Geometry: final body of the model. Coordinates: model frame, mm. A direction names the side the tool comes from. Give positions to 0.01 mm unless a question says otherwise; leave off trailing zeros. Write each loop counter-clockwise with the first axis right and the second up, starting at its lowest first coordinate (ties: lowest second). Pieces come first, ordered by that corner, then holes. Notation, with made-up numbers: (75.5, 89.5) - (101.5, 89.5) arc R13 cw to (101.5, 96.5) - close; hole circle Ø10 at (56.5, 62.5). An arc over 180 degrees is marked (long way). Return JSON: item names as keys, results as strings.
from build123d import *

# Parameters (mm, degrees)
SKETCH1_R           = 1.5
SKETCH1_W           = 23
SKETCH1_H           = 12
BOSS_EXTRUDE1_DEPTH = 5
FILLET1_R           = 5
FILLET2_R           = 5
FILLET3_R           = 5
FILLET4_R           = 5
FILLET5_R           = 5
FILLET6_R           = 5


with BuildPart() as part:
    # Sketch1 → Boss-Extrude1 (new body)
    with BuildSketch(Plane.XY):
        Polygon((28.231059773, 10.187376726), (15.644565305, 25.187376726), (-9.182445759, 25.187376726), (-21.768940227, 10.187376726), (-21.768940227, -14.812623274), (-16.768940227, -14.812623274), (-16.768940227, -9.812623274), (-11.768940227, -9.812623274), (-11.768940227, -14.812623274), (-4.768940227, -14.812623274), (-4.768940227, -9.812623274), (11.231059773, -9.812623274), (11.231059773, -14.812623274), (18.231059773, -14.812623274), (18.231059773, -9.812623274), (23.231059773, -9.812623274), (23.231059773, -14.812623274), (28.231059773, -14.812623274), align=None)
        with Locations((-2.768940227, 22.187376726)):
            Circle(SKETCH1_R, mode=Mode.SUBTRACT)
        with Locations((9.231059773, 22.187376726)):
            Circle(SKETCH1_R, mode=Mode.SUBTRACT)
        with Locations((-6.361893004, 3.645929715)):
            Circle(SKETCH1_R, mode=Mode.SUBTRACT)
        with Locations((11.531059773, 3.445929715)):
            Rectangle(SKETCH1_W, SKETCH1_H, mode=Mode.SUBTRACT)
    extrude(amount=BOSS_EXTRUDE1_DEPTH)

    # Fillet1
    fillet1_edges = [part.edges().sort_by_distance(p)[0] for p in [
        (15.644565305, 25.187376726, 2.5),
    ]]
    fillet(fillet1_edges, radius=FILLET1_R)

    # Fillet2
    fillet2_edges = [part.edges().sort_by_distance(p)[0] for p in [
        (28.231059773, 10.187376726, 2.5),
    ]]
    fillet(fillet2_edges, radius=FILLET2_R)

    # Fillet3
    fillet3_edges = [part.edges().sort_by_distance(p)[0] for p in [
        (28.231059773, -14.812623274, 2.5),
    ]]
    fillet(fillet3_edges, radius=FILLET3_R - 0.0001)  # a hair under: the kernel refuses the full size

    # Fillet4
    fillet4_edges = [part.edges().sort_by_distance(p)[0] for p in [
        (-9.182445759, 25.187376726, 2.5),
    ]]
    fillet(fillet4_edges, radius=FILLET4_R)

    # Fillet5
    fillet5_edges = [part.edges().sort_by_distance(p)[0] for p in [
        (-21.768940227, 10.187376726, 2.5),
    ]]
    fillet(fillet5_edges, radius=FILLET5_R)

    # Fillet6
    fillet6_edges = [part.edges().sort_by_distance(p)[0] for p in [
        (-21.768940227, -14.812623274, 2.5),
    ]]
    fillet(fillet6_edges, radius=FILLET6_R - 0.0001)  # a hair under: the kernel refuses the full size


solid = part.part
Q1. Section query B-B, the plane x = 6. Return the cut outline in (y, z).
Answer key:
{"outline": "(-9.81, 0) - (-2.55, 0) - (-2.55, 5) - (-9.81, 5) - close; (9.45, 0) - (25.19, 0) - (25.19, 5) - (9.45, 5) - close"}
Q2. Set-up query: faces 1 (the flat face through (-21.769, -1, 2)), 2 (the flat face through (11.231, -12, 2)), 3 (the flat face through (23.031, 3, 2)). Return all of +Z, -Z, +X, -X, +Y, -Y with unobstructed straight access to the full face (end or side cutting, diameter ignored); none if empty.
Answer key:
{"face 1": "+Z, -Z, -X, +Y, -Y", "face 2": "+Z, -Z, -Y", "face 3": "+Z, -Z"}
Q3. Mould query, pull axis X, two halves, no side actions, for faces 4 (the flat face through (15, -14.813, 2)), 5 (the cylindrical face through (27.92, 10.1, 2.54)), 6 (the flat face through (3, -9.813, 2)). Classes: pulls with the +X half, pulls with the -X half, needs draft (parallel to the pull), parting line crosses it, or undercut.
Answer key:
{"face 4": "needs draft", "face 5": "pulls with the +X half", "face 6": "undercut"}
Q4. Section query A-A, the plane y = -1.5. Return the cut outline in (x, z).
Answer key:
{"outline": "(-21.77, 0) - (0.03, 0) - (0.03, 5) - (-21.77, 5) - close; (23.03, 0) - (28.23, 0) - (28.23, 5) - (23.03, 5) - close"}
Q5. Pin query (flat end, axial travel): P1, Ø2.5, axis at y = -13, z = 3.5, coming from the +X side; P2, Ø1.5, axis at x = 22, z = 2.5, coming from the -Y side; P3, Ø1.5, axis at y = -11.5, z = 1.5, coming from the -X side; P4, Ø1.8, axis at x = 9.23, y = 22.19, coming from the -Z side. Return the tip coordinate at first contact, or that it passes through.
Answer key:
{"P1": "stops at x = 27.84", "P2": "stops at y = -9.81", "P3": "stops at x = -21.68", "P4": "passes through"}
Q6. Section query C-C, the plane z = 1.7. Count the separate pieces of the cut face and the enclosed holes in it, plus the area to 3 significant figures.
Answer key:
{"separate pieces": "1", "enclosed holes": "4", "area": "1,370 mm^2"}
Q7. Section query D-D, the plane x = -0.5. Return the cut outline in (y, z).
Answer key:
{"outline": "(-9.81, 0) - (25.19, 0) - (25.19, 5) - (-9.81, 5) - close"}
Q8. Material intervals for probe 1 along Y at (x, z) = (1, 1.15); probe 2 along X at (y, z) = (3, 4.85); probe 3 along X at (y, z) = (1, 4.55), sorted ascending. Write a range as [from, to].
Answer key:
{"probe 1": "y = [-9.81, -2.55], [9.45, 25.19]", "probe 2": "x = [-21.77, -7.72], [-5.01, 0.03], [23.03, 28.23]", "probe 3": "x = [-21.77, 0.03], [23.03, 28.23]"}
